Here's how the part is built. I have some questions about the finished solid (model axes, mm). Round coordinates to 2 decimals unless told otherwise and drop trailing zeros. Order: outer loops, then holes, each group sorted by start corner. A loop starts at its lowest first (then second) coordinate and runs counter-clockwise, first axis right, second up. Notation, with made-up numbers: (-5, 5.25) - (14, 5.25) arc R20 cw to (14, 27.25) - close; hole circle Ø7 at (-40, -4.75). An arc over 180 degrees is marked (long way). Answer as a JSON object with one key per item and string values.
```python
from build123d import *

# Parameters (mm, degrees)
SKETCH1_R             = 18.415
BOSS_EXTRUDE1_DEPTH   = 3.175
CIRPATTERN1_COUNT     = 6
F_2_56_TAPPED_HOLE1_D = 1.778
CHAMFER1_SIZE         = 1.27


with BuildPart() as part:
    # Sketch1 → Boss-Extrude1 (new body)
    with BuildSketch(Plane.XY):
        Circle(SKETCH1_R)
    extrude(amount=BOSS_EXTRUDE1_DEPTH)

    # Sketch3 → Cut-Revolve1 (revolve, cut)
    with BuildSketch(Plane(origin=(0, 0, 0), x_dir=(0, 0, -1), z_dir=(1, 0, 0))):
        with BuildLine():
            Line((-6.01345, 8.255), (-0.84455, 8.255))
            ThreePointArc((-0.84455, 8.255), (-3.429, 10.83945), (-6.01345, 8.255))
        make_face()
    cut_revolve1 = revolve(axis=Axis((0, 8.255, 6.01345), (0, 0, -1)), mode=Mode.SUBTRACT)

    # CirPattern1: Cut-Revolve1 ×6 about axis
    cirpattern1_axis = Axis((0, 0, 0), (0, 0, 1))
    for i in range(1, CIRPATTERN1_COUNT):
        add(cut_revolve1.rotate(cirpattern1_axis, i * 360 / CIRPATTERN1_COUNT), mode=Mode.SUBTRACT)

    # 2-56 Tapped Hole1 (through all)
    with Locations(Plane(origin=(0, 0, 0), x_dir=(-1, 0, 0), z_dir=(0, 0, -1))):
        with Locations((0, 15.24), (15.24, 0), (0, -15.24), (-15.24, 0)):
            Hole(F_2_56_TAPPED_HOLE1_D / 2)

    # Chamfer1
    chamfer1_edges = [part.edges().sort_by_distance(p)[0] for p in [
        (-18.415, 0, 3.175),
    ]]
    chamfer(chamfer1_edges, length=CHAMFER1_SIZE)


solid = part.part
```
1. Imagine slicing it at C-C (z = 2.55). Give the number of separate pieces and of enclosed holes in the cut face, plus the area to 3 significant figures.
Responses:
{"separate pieces": "1", "enclosed holes": "10", "area": "871 mm2"}
2. If I drill on L1, parallel to Y at x = 0, z = 0.3 (3 decimals); L2, parallel to Y at x = 15.24, z = 2.4; L3, parallel to X at y = -9, z = 2.55, over which ranges is the centre line in solid material (lowest first)? Write a range as [from, to].
Responses:
{"L1": "[-18.415, -16.129], [-14.351, 14.351], [16.129, 18.415]", "L2": "[-9.43, -0.89], [0.89, 9.43]", "L3": "[-15.32, -2.31], [2.31, 15.32]"}
3. For P1, Ø1.5, axis at x = -6, z = 1.5, coming from the -Y side; P2, Ø1, axis at x = 13.5, z = 0.5, coming from the +Y side, each with a flat end and sliding along its axis, tell me the tip position at first contact or that it passes through.
Responses:
{"P1": "y = -17.65", "P2": "y = 13.04"}
4. Imagine slicing it at A-A (x = 0). List the corners of the cut face in (y, z) for me (3 decimals).
Responses:
{"outline": "(-18.415, 0) - (-16.129, 0) - (-16.129, 3.175) - (-17.145, 3.175) - (-18.415, 1.905) - close; (-14.351, 0) - (14.351, 0) - (14.351, 3.175) - (10.827, 3.175) arc R2.584 cw to (5.683, 3.175) - (-5.683, 3.175) arc R2.584 cw to (-10.827, 3.175) - (-14.351, 3.175) - close; (16.129, 0) - (18.415, 0) - (18.415, 1.905) - (17.145, 3.175) - (16.129, 3.175) - close"}
5. Thinking about a two-plate mould opening in X: for faces 1 (the face through (0, 0, 3.175)), 2 (the face through (-0.12, 16.12, 1.61)), 3 (the face through (-14.61, -11.21, 0.94)), which applies, pulls with the +X half, pulls with the -X half, needs draft (parallel to the pull), parting line crosses it, or undercut?
Responses:
{"face 1": "needs draft", "face 2": "undercut", "face 3": "parting line crosses it"}
6. Imagine slicing it at B-B (y = 0). List the corners of the cut face in (x, z) for me (3 decimals), plus the area to 3 significant figures.
Responses:
{"outline": "(-18.415, 0) - (-16.129, 0) - (-16.129, 3.175) - (-17.145, 3.175) - (-18.415, 1.905) - close; (-14.351, 0) - (14.351, 0) - (14.351, 3.175) - (-14.351, 3.175) - close; (16.129, 0) - (18.415, 0) - (18.415, 1.905) - (17.145, 3.175) - (16.129, 3.175) - close", "area": "104 mm2"}
